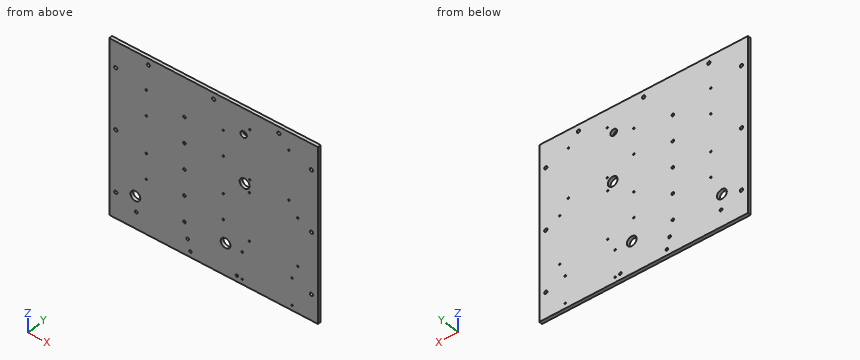
from build123d import *

# Parameters (mm, degrees)
SKETCH1_W           = 406.4
SKETCH1_H           = 342.9
BOSS_EXTRUDE1_DEPTH = 6.35
SKETCH3_R           = 3.175
CUT_EXTRUDE1_DEPTH  = 532.772218624
SKETCH4_R           = 9.525
SKETCH4_R_2         = 1.5875
SKETCH4_R_3         = 2.5
SKETCH4_R_4         = 2.667
SKETCH4_R_5         = 2.54
SKETCH4_R_6         = 1.5
SKETCH4_R_7         = 6.35
CUT_EXTRUDE2_DEPTH  = 532.772218624


with BuildPart() as part:
    # Sketch1 → Boss-Extrude1 (new body)
    with BuildSketch(Plane(origin=(0, 0, 0), x_dir=(1, 0, 0), z_dir=(0, 1, 0))):
        with Locations((203.2, 171.45)):
            Rectangle(SKETCH1_W, SKETCH1_H)
    extrude(amount=BOSS_EXTRUDE1_DEPTH)

    # Sketch3 → Cut-Extrude1 (cut, through all)
    with BuildSketch(Plane(origin=(0, 6.35, 0), x_dir=(1, 0, 0), z_dir=(0, 1, 0))):
        with Locations(Location((203.2, 12.7, 0), (0, 0, 270))):
            Circle(SKETCH3_R)
        with Locations(Location((330.2, 12.7, 0), (0, 0, 270))):
            Circle(SKETCH3_R)
        with Locations(Location((76.2, 12.7, 0), (0, 0, 270))):
            Circle(SKETCH3_R)
        with Locations(Location((12.7, 171.45, 0), (0, 0, 270))):
            Circle(SKETCH3_R)
        with Locations(Location((393.7, 171.45, 0), (0, 0, 270))):
            Circle(SKETCH3_R)
        with Locations(Location((12.7, 292.1, 0), (0, 0, 270))):
            Circle(SKETCH3_R)
        with Locations(Location((12.7, 50.8, 0), (0, 0, 270))):
            Circle(SKETCH3_R)
        with Locations(Location((393.7, 50.8, 0), (0, 0, 270))):
            Circle(SKETCH3_R)
        with Locations(Location((393.7, 292.1, 0), (0, 0, 270))):
            Circle(SKETCH3_R)
    extrude(amount=-CUT_EXTRUDE1_DEPTH, mode=Mode.SUBTRACT)

    # Sketch4 → Cut-Extrude2 (cut, through all)
    with BuildSketch(Plane(origin=(0, 6.35, 0), x_dir=(1, 0, 0), z_dir=(0, 1, 0))):
        with Locations(Location((226.4, 279.9, 0), (0, 0, 270))):
            Circle(SKETCH4_R)
        with Locations(Location((50.8, 279.9, 0), (0, 0, 270))):
            Circle(SKETCH4_R)
        with Locations(Location((222.1748, 63.265, 0), (0, 0, 270))):
            Circle(SKETCH4_R_2)
        with Locations(Location((222.1748, 113.265, 0), (0, 0, 270))):
            Circle(SKETCH4_R_2)
        with Locations(Location((72.1748, 113.265, 0), (0, 0, 270))):
            Circle(SKETCH4_R_2)
        with Locations(Location((72.1748, 63.265, 0), (0, 0, 270))):
            Circle(SKETCH4_R_2)
        with Locations(Location((72.1748, 186.295, 0), (0, 0, 270))):
            Circle(SKETCH4_R_2)
        with Locations(Location((72.1748, 236.295, 0), (0, 0, 270))):
            Circle(SKETCH4_R_2)
        with Locations(Location((222.1748, 236.295, 0), (0, 0, 270))):
            Circle(SKETCH4_R_2)
        with Locations(Location((222.1748, 186.295, 0), (0, 0, 270))):
            Circle(SKETCH4_R_2)
        with Locations(Location((248.4501, 331.47, 0), (0, 0, 270))):
            Circle(SKETCH4_R_3)
        with Locations(Location((157.9499, 331.47, 0), (0, 0, 270))):
            Circle(SKETCH4_R_3)
        with Locations(Location((52.5398, 309.88, 0), (0, 0, 270))):
            Circle(SKETCH4_R_4)
        with Locations(Location((152.5398, 309.88, 0), (0, 0, 270))):
            Circle(SKETCH4_R_4)
        with Locations(Location((146.3548, 178.4985, 0), (0, 0, 270))):
            Circle(SKETCH4_R_5)
        with Locations(Location((146.3548, 127.6985, 0), (0, 0, 270))):
            Circle(SKETCH4_R_5)
        with Locations(Location((146.3548, 76.8985, 0), (0, 0, 270))):
            Circle(SKETCH4_R_5)
        with Locations(Location((146.3548, 280.0985, 0), (0, 0, 270))):
            Circle(SKETCH4_R_5)
        with Locations(Location((146.3548, 229.2985, 0), (0, 0, 270))):
            Circle(SKETCH4_R_5)
        with Locations(Location((355.833, 333.05, 0), (0, 0, 270))):
            Circle(SKETCH4_R_6)
        with Locations(Location((258.833, 333.05, 0), (0, 0, 270))):
            Circle(SKETCH4_R_6)
        with Locations(Location((355.833, 280.05, 0), (0, 0, 270))):
            Circle(SKETCH4_R_6)
        with Locations(Location((258.833, 280.05, 0), (0, 0, 270))):
            Circle(SKETCH4_R_6)
        with Locations(Location((366.9502, 251.78, 0), (0, 0, 270))):
            Circle(SKETCH4_R_6)
        with Locations(Location((272.9502, 251.78, 0), (0, 0, 270))):
            Circle(SKETCH4_R_6)
        with Locations(Location((366.9502, 157.78, 0), (0, 0, 270))):
            Circle(SKETCH4_R_6)
        with Locations(Location((272.9502, 157.78, 0), (0, 0, 270))):
            Circle(SKETCH4_R_6)
        with Locations(Location((349.7002, 35.25, 0), (0, 0, 270))):
            Circle(SKETCH4_R_6)
        with Locations(Location((349.7002, 132.25, 0), (0, 0, 270))):
            Circle(SKETCH4_R_6)
        with Locations(Location((273.7002, 132.25, 0), (0, 0, 270))):
            Circle(SKETCH4_R_6)
        with Locations(Location((273.7002, 35.25, 0), (0, 0, 270))):
            Circle(SKETCH4_R_6)
        with Locations(Location((263.4, 145, 0), (0, 0, 270))):
            Circle(SKETCH4_R)
        with Locations(Location((261.4925, 50.8, 0), (0, 0, 270))):
            Circle(SKETCH4_R_7)
    extrude(amount=-CUT_EXTRUDE2_DEPTH, mode=Mode.SUBTRACT)


solid = part.part
Build history of the part. All positions in model axes, mm. Round coordinates to 2 decimals unless told otherwise and drop trailing zeros. Write each loop counter-clockwise with the first axis right and the second up, starting at its lowest first coordinate (ties: lowest second). Pieces come first, ordered by that corner, then holes. Notation, with made-up numbers: M -0.5,67 L 4.5,67 A22 ccw 4.5,106 Z; hole C 84,-11.75 d1. An arc over 180 degrees is marked long. Answer as a JSON object with one key per item and string values. Group by question number.
(1) Flat gauge pin, fed straight in: pin 1 (17 mm diameter, centred on x = 226.4, z = -279.9, fed in from +Y). Where does the tip first touch, or does it go through?
(2) Drill centre lines: L1, parallel to Z at x = 349.5, y = 1.75; L2, parallel to X at y = 3, z = -171.45 (3 decimals); L3, parallel to X at y = 4.75, z = -50.8 (1 decimal). Where is each one in solid material? Low to high.
(3) Cut at A-A (z = -145). Give the cut face in (x, y) (3 decimals), and give its area (3 significant figures).
Responses:
{
 "1": {"pin 1": "passes through"},
 "2": {"L1": "z = -342.9 to -133.74, -130.76 to -36.74, -33.76 to 0", "L2": "x = 0 to 9.525, 15.875 to 390.525, 396.875 to 406.4", "L3": "x = 0 to 9.5, 15.9 to 255.1, 267.8 to 390.5, 396.9 to 406.4"},
 "3": {"outline": "M 0,0 L 253.875,0 L 253.875,6.35 L 0,6.35 Z; M 272.925,0 L 406.4,0 L 406.4,6.35 L 272.925,6.35 Z", "area": "2,460 mm2"}
}
